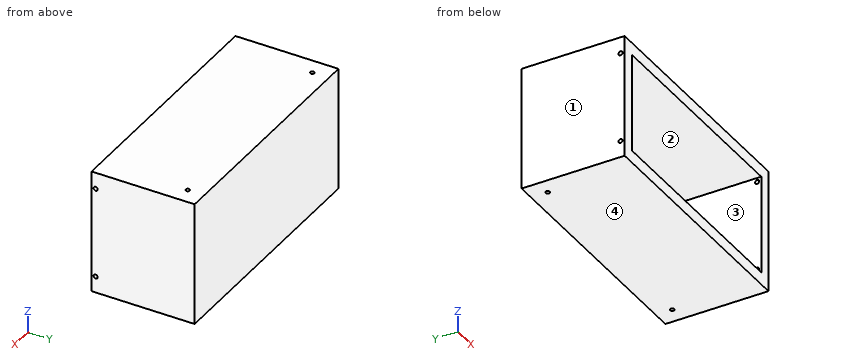
from build123d import *

# Parameters (mm, degrees)
SKETCH1_W           = 300
SKETCH1_H           = 150
BOSS_EXTRUDE1_DEPTH = 125
SKETCH2_W           = 270
SKETCH2_H           = 120
CUT_EXTRUDE1_DEPTH  = 110
SKETCH4_R           = 2.5
CUT_EXTRUDE5_DEPTH  = 350
SKETCH6_R           = 2.5
CUT_EXTRUDE6_DEPTH  = 175


with BuildPart() as part:
    # Sketch1 → Boss-Extrude1 (new body)
    with BuildSketch(Plane(origin=(0, 0, 0), x_dir=(1, 0, 0), z_dir=(0, 1, 0))):
        Rectangle(SKETCH1_W, SKETCH1_H)
    extrude(amount=BOSS_EXTRUDE1_DEPTH)

    # Sketch2 → Cut-Extrude1 (cut)
    with BuildSketch(Plane.XZ):
        Rectangle(SKETCH2_W, SKETCH2_H)
    extrude(amount=-CUT_EXTRUDE1_DEPTH, mode=Mode.SUBTRACT)

    # Sketch4 → Cut-Extrude5 (cut)
    with BuildSketch(Plane(origin=(150, 0, 0), x_dir=(0, 0, -1), z_dir=(1, 0, 0))):
        with Locations((-55, 5)):
            Circle(SKETCH4_R)
        with Locations((55, 5)):
            Circle(SKETCH4_R)
    extrude(amount=-CUT_EXTRUDE5_DEPTH, mode=Mode.SUBTRACT)

    # Sketch6 → Cut-Extrude6 (cut)
    with BuildSketch(Plane.XY.offset(75)):
        with Locations((-130, 105)):
            Circle(SKETCH6_R)
        with Locations((130, 105)):
            Circle(SKETCH6_R)
    extrude(amount=-CUT_EXTRUDE6_DEPTH, mode=Mode.SUBTRACT)


solid = part.part
Verification items for the finished model (mm, model axes). Face numbers are marked on the shaded views. Coordinates: 2 decimals unless noted, no trailing zeros. Loops run counter-clockwise (first coordinate to the right, second up) from the corner with the lowest first, then second, coordinate; pieces in that order, holes last. Notation, with made-up numbers: M 87,50 L 103,50 A36 cw 103,86 Z; hole C 51,-18 d4. An arc over 180 degrees is marked long. One line per item, written item: value.
1. Section check B-B on y = 21.5. Record the cut outline in (x, z).
Answers follow:
outline: M -150,-75 L 150,-75 L 150,75 L -150,75 Z; hole M -135,-60 L 135,-60 L 135,60 L -135,60 Z
2. Gauge pin test, flat ends, axial feed: P1, Ø8, axis at x = -79.5, z = -30, coming from the -Y side; P2, Ø4.5, axis at y = 5, z = 55, coming from the -X side. Record the tip position at first contact, or that the pin passes through.
Answers follow:
P1: y = 110
P2: through
3. Mould release check, pull along X, two halves, no side actions. Record for the marked faces 1, 2, 3 and 4: pulls with the +X half, pulls with the -X half, needs draft (parallel to the pull), parting line crosses it, or undercut.
Answers follow:
face 1: pulls with the -X half
face 2: undercut
face 3: undercut
face 4: needs draft
4. Section check A-A on x = -119.5. Record the cut outline in (y, z).
Answers follow:
outline: M 0,-75 L 125,-75 L 125,75 L 0,75 L 0,60 L 110,60 L 110,-60 L 0,-60 Z
5. Section check C-C on z = 49. Record the cut outline in (x, y).
Answers follow:
outline: M -150,0 L -135,0 L -135,110 L 135,110 L 135,0 L 150,0 L 150,125 L -150,125 Z
6. Material ranges on line 1 along Z through (x, y) = (-87.5, 90.5); line 2 along Y through (x, z) = (130, -66); line 3 along X through (y, z) = (64, -25.5), recorded low to high. Write a range as from..to.
Answers follow:
line 1: -75..-60, 60..75
line 2: 0..102.5, 107.5..125
line 3: -150..-135, 135..150
